For this review, use the dimensioned drawing (mm, ordinates from the lowest corner) and the shaded views. A direction names the side the tool comes from. Round coordinates to 2 decimals unless told otherwise and drop trailing zeros. Order: outer loops, then holes, each group sorted by start corner. A loop starts at its lowest first (then second) coordinate and runs counter-clockwise, first axis right, second up. Notation, with made-up numbers: M 82,88.5 L 93,88.5 A22 cw 93,118.5 Z; hole C -2,-28 d7. An arc over 180 degrees is marked long. Use a Markdown table: item, result. Add a question column.
1. To check wall thickness, follow probe 1 along X at (y, z) = (10, 4.55); probe 2 along X at (y, z) = (22, 4.2). State the ranges of each line that lie inside material, in increasing order.
2. Consider section B-B on x = 22. State the section outline as (y, z) points.
3. Consider section A-A on z = 3.6. Count the separate pieces of the cut face and the enclosed holes in it, then the cut area to 3 significant figures.
4. Consider section C-C on y = 25. State the section outline as (x, z) points.
5. Insertion check: P1, Ø5, axis at x = 27, y = 39.5, coming from the +Z side. The pin has a flat end and moves straight along its axis. Give the tip position at first contact, or say it passes through.
6. For the marked faces 3 and 4, list the 3-axis set-ups (+Z, -Z, +X, -X, +Y, -Y) from which the entire face can be reached by the end or side of a thin tool; tool diameter is ignored.
7. The part is to be moulded in two halves that separate along X. For the marked faces 1 and 2, say which applies: +X half, -X half, draft (parallel to the pull), parting line (faces both ways), or undercut.
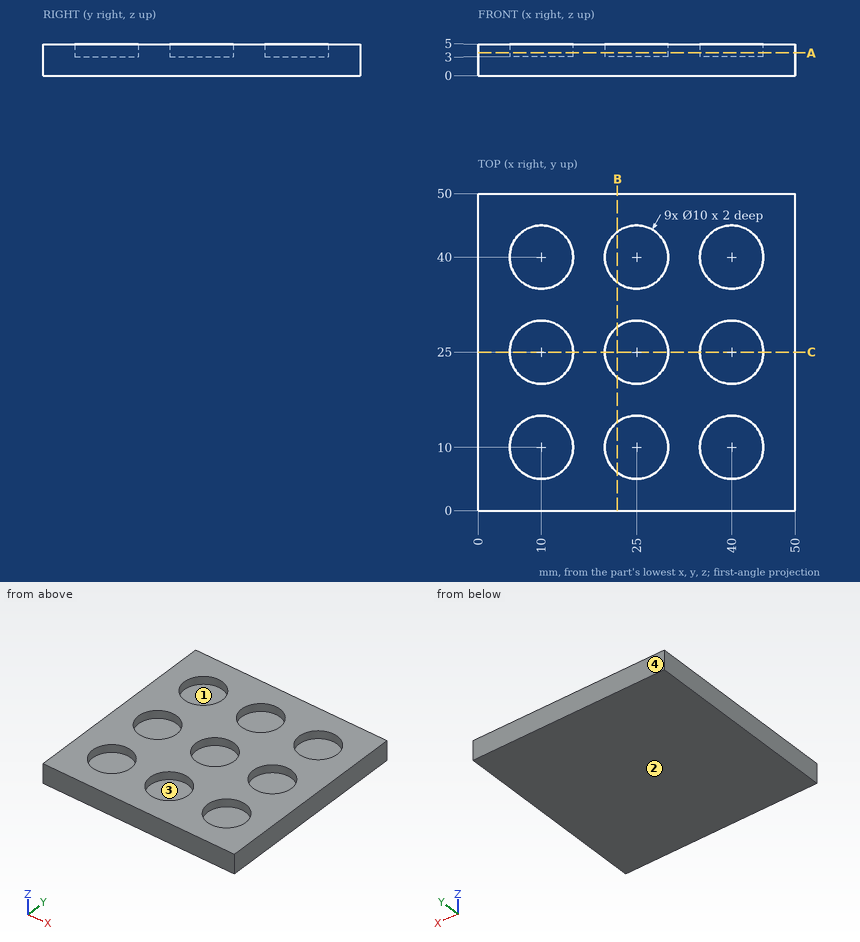
Answer block:
| question | item | result |
|---|---|---|
| 1 | probe 1 | 0 to 5, 15 to 20, 30 to 35, 45 to 50 |
| 1 | probe 2 | 0 to 6, 14 to 21, 29 to 36, 44 to 50 |
| 2 | outline | M 0,0 L 50,0 L 50,5 L 44,5 L 44,3 L 36,3 L 36,5 L 29,5 L 29,3 L 21,3 L 21,5 L 14,5 L 14,3 L 6,3 L 6,5 L 0,5 Z |
| 3 | separate pieces | 1 |
| 3 | enclosed holes | 9 |
| 3 | area | 1,790 mm^2 |
| 4 | outline | M 0,0 L 50,0 L 50,5 L 45,5 L 45,3 L 35,3 L 35,5 L 30,5 L 30,3 L 20,3 L 20,5 L 15,5 L 15,3 L 5,3 L 5,5 L 0,5 Z |
| 5 | P1 | z = 3 |
| 6 | face 3 | +Z |
| 6 | face 4 | +Z, -Z, +X, -X, +Y |
| 7 | face 1 | undercut |
| 7 | face 2 | draft |
